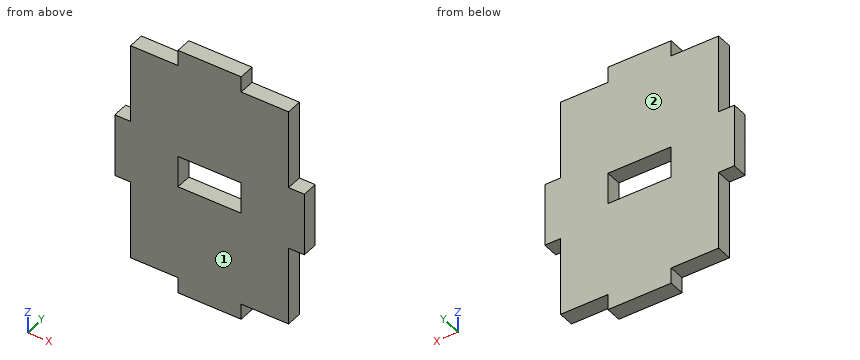
```python
from build123d import *

# Parameters (mm, degrees)
F1_DEPTH = 5
F2_W     = 20
F2_H     = 10
F3_DEPTH = 25


with BuildPart() as f1:
    # F0 (on Front) → F1 (new body)
    with BuildSketch(Plane.XZ):
        Polygon((0, 25), (0, 0), (15, 0), (15, -5), (35, -5), (35, 0), (50, 0), (50, 25), (55, 25), (55, 45), (50, 45), (50, 70), (35, 70), (35, 75), (15, 75), (15, 70), (0, 70), (0, 45), (-5, 45), (-5, 25), align=None)
    extrude(amount=F1_DEPTH)

    # F2 (on face) → F3 (cut)
    with BuildSketch(Plane.XZ.offset(5)):
        with Locations((25, 35)):
            Rectangle(F2_W, F2_H)
    extrude(amount=-F3_DEPTH, mode=Mode.SUBTRACT)


solid = f1.part
```
Part model, mm, in its own coordinate system. Face numbers are marked on the shaded views. Round coordinates to 2 decimals unless told otherwise and drop trailing zeros. Loops run counter-clockwise (first coordinate to the right, second up) from the corner with the lowest first, then second, coordinate; pieces in that order, holes last. Notation, with made-up numbers: (11.5, 17) -> (61.5, 17) arc R13 cw to (61.5, 37) -> close; hole circle Ø1 at (18, 82). An arc over 180 degrees is marked (long way). Use one line per item in the form item = value. Start each with the question number.
Item 1: Band-saw the part on A-A (x = 23.5). List the corners of the cut face in (y, z).
Item 2: Band-saw the part on D-D (x = 51.5). List the corners of the cut face in (y, z).
Item 3: Drill centre lines: line 1 along X through (y, z) = (-3.3, 38); line 2 along Z through (x, y) = (34.5, -2); line 3 along Z through (x, y) = (1, -0.4). Where is each one in solid material? Low to high.
Item 4: Two-plate mould, pull along Y, no slides. Class the marked faces 1 and 2: released by +Y, released by -Y, zero draft, split by the parting line, or undercut.
Item 5: Band-saw the part on B-B (z = 37). List the corners of the cut face in (x, y).
Item 6: Drop flat-ended pins along their axis: pin 1 Ø2.5 at (x, y) = (7, -1.5) entering from -Z; pin 2 Ø2.5 at (x, y) = (-2, -2) entering from -Z; pin 3 Ø1.5 at (x, y) = (42.5, -2) entering from +Z; pin 4 Ø3 at (x, z) = (17.5, 6) entering from +Y. Give the stop position or say it passes through.
Item 7: Band-saw the part on C-C (y = -2). List the corners of the cut face in (x, z), plus the area to 3 significant figures.
Data:
q1.outline = (-5, -5) -> (0, -5) -> (0, 30) -> (-5, 30) -> close; (-5, 40) -> (0, 40) -> (0, 75) -> (-5, 75) -> close
q2.outline = (-5, 25) -> (0, 25) -> (0, 45) -> (-5, 45) -> close
q3.line_1 = -5 to 15, 35 to 55
q3.line_2 = -5 to 30, 40 to 75
q3.line_3 = 0 to 70
q4.face_1 = released by -Y
q4.face_2 = released by +Y
q5.outline = (-5, -5) -> (15, -5) -> (15, 0) -> (-5, 0) -> close; (35, -5) -> (55, -5) -> (55, 0) -> (35, 0) -> close
q6.pin_1 = 0
q6.pin_2 = 25
q6.pin_3 = 70
q6.pin_4 = 0
q7.outline = (-5, 25) -> (0, 25) -> (0, 0) -> (15, 0) -> (15, -5) -> (35, -5) -> (35, 0) -> (50, 0) -> (50, 25) -> (55, 25) -> (55, 45) -> (50, 45) -> (50, 70) -> (35, 70) -> (35, 75) -> (15, 75) -> (15, 70) -> (0, 70) -> (0, 45) -> (-5, 45) -> close; hole (15, 30) -> (35, 30) -> (35, 40) -> (15, 40) -> close
q7.area = 3,700 mm^2
